```python
from build123d import *

# Parameters (mm, degrees)
SKETCH1_W           = 70
SKETCH1_H           = 100
BOSS_EXTRUDE1_DEPTH = 50
SKETCH3_W           = 68
SKETCH3_H           = 97.5
CUT_EXTRUDE1_DEPTH  = 45
SKETCH5_W           = 30
SKETCH5_H           = 40
CUT_EXTRUDE2_DEPTH  = 5.5


with BuildPart() as part:
    # Sketch1 → Boss-Extrude1 (new body)
    with BuildSketch(Plane(origin=(0, 0, 0), x_dir=(1, 0, 0), z_dir=(0, 1, 0))):
        Rectangle(SKETCH1_W, SKETCH1_H)
    extrude(amount=BOSS_EXTRUDE1_DEPTH)

    # Sketch3 → Cut-Extrude1 (cut)
    with BuildSketch(Plane(origin=(0, 50, 0), x_dir=(1, 0, 0), z_dir=(0, 1, 0))):
        Rectangle(SKETCH3_W, SKETCH3_H)
    extrude(amount=-CUT_EXTRUDE1_DEPTH, mode=Mode.SUBTRACT)

    # Sketch5 → Cut-Extrude2 (cut)
    with BuildSketch(Plane(origin=(0, 0, -50), x_dir=(-1, 0, 0), z_dir=(0, 0, -1))):
        with Locations((15, 35.461610705)):
            Rectangle(SKETCH5_W, SKETCH5_H)
    extrude(amount=-CUT_EXTRUDE2_DEPTH, mode=Mode.SUBTRACT)


solid = part.part
```
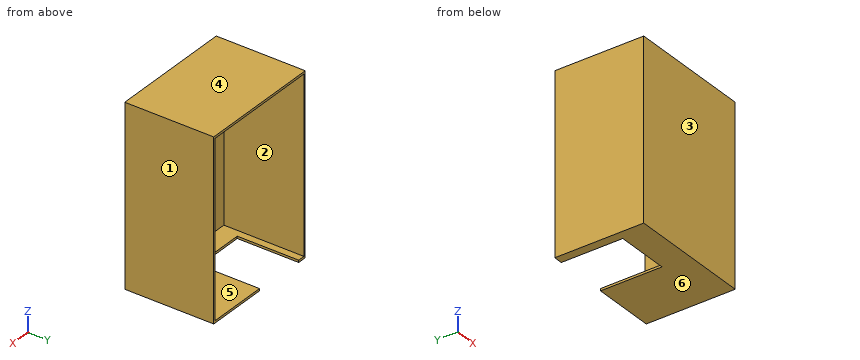
For this review, take the finished solid that the model builds, in its own axes (mm). Face numbers are marked on the shaded views. A direction names the side the tool comes from. Coordinates: 2 decimals unless noted, no trailing zeros. Loops run counter-clockwise (first coordinate to the right, second up) from the corner with the lowest first, then second, coordinate; pieces in that order, holes last. Notation, with made-up numbers: (54, 43) - (101, 43) arc R21 cw to (101, 66) - close; hole circle Ø3 at (-19.75, -30.5). An arc over 180 degrees is marked (long way). Use one line per item in the form item = value. Start each with the question number.
1) Take a section at C-C (z = 30). State the section outline as (x, y) points, plus the area to 3 significant figures.
2) Take a section at A-A (y = 10). State the section outline as (x, z) points, plus the area to 3 significant figures.
3) Take a section at B-B (x = 12). State the section outline as (y, z) points, plus the area to 4 significant figures.
4) Take a section at D-D (y = 17). State the section outline as (x, z) points.
5) For pin 1 (4 mm diameter, centred on x = 24.5, z = -12.5, fed in from +Y), flat-tipped, find the tip position at first contact; note if it passes through.
6) Draft analysis for pull direction Z (two halves, no side actions). For the marked faces 3, 4, 5 and 6, state which applies: released by +Z, released by -Z, zero draft, split by the parting line, or undercut.
7) For the marked faces 1 and 2, list the 3-axis set-ups (+Z, -Z, +X, -X, +Y, -Y) from which the entire face can be reached by the end or side of a thin tool; tool diameter is ignored.
8) To check wall thickness, follow probe 1 along X at (y, z) = (32, -45.5); probe 2 along Z at (x, y) = (5, 47.5); probe 3 along Y at (x, z) = (-7.5, 18). State the ranges of each line that lie inside material, in increasing order. Write a range as from..to.
From the geometry:
q1.outline = (-35, 0) - (35, 0) - (35, 50) - (34, 50) - (34, 5) - (-34, 5) - (-34, 50) - (-35, 50) - close
q1.area = 440 mm2
q2.outline = (-35, -50) - (35, -50) - (35, 50) - (-35, 50) - close; hole (-34, -48.75) - (34, -48.75) - (34, 48.75) - (-34, 48.75) - close
q2.area = 370 mm2
q3.outline = (0, -50) - (50, -50) - (50, -48.75) - (5, -48.75) - (5, 48.75) - (50, 48.75) - (50, 50) - (0, 50) - close
q3.area = 612.5 mm2
q4.outline = (-35, -50) - (-30, -50) - (-30, -48.75) - (-34, -48.75) - (-34, 48.75) - (34, 48.75) - (34, -48.75) - (0, -48.75) - (0, -50) - (35, -50) - (35, 50) - (-35, 50) - close
q5.pin_1 = 5
q6.face_3 = zero draft
q6.face_4 = released by +Z
q6.face_5 = undercut
q6.face_6 = released by -Z
q7.face_1 = +Z, -Z, +X, +Y, -Y
q7.face_2 = +Y
q8.probe_1 = -35..-34, 34..35
q8.probe_2 = -50..-48.75, 48.75..50
q8.probe_3 = 0..5
